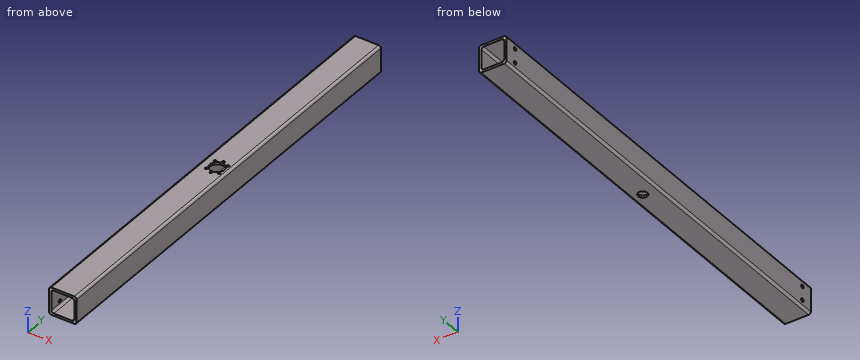
```python
from build123d import *

# Parameters (mm, degrees)
F1_DEPTH = 1226
F2_R     = 5
F3_DEPTH = 25.4
F4_R     = 3.3
F4_R_2   = 20.25
F5_DEPTH = 76.201
F6_W     = 51.969446
F6_H     = 157.89732
F6_R     = 13
F7_DEPTH = 6.35


with BuildPart() as f1:
    # F0 (on Front) → F1 (new body)
    with BuildSketch(Plane.XZ):
        with BuildLine():
            Line((50.800001, 36.691132), (-12.699999, 36.691132))
            ThreePointArc((-12.699999, 36.691132), (-17.190127, 34.83126), (-19.049999, 30.341132))
            Line((-19.049999, 30.341132), (-19.049999, -33.158868))
            ThreePointArc((-19.049999, -33.158868), (-17.190127, -37.648996), (-12.699999, -39.508868))
            Line((-12.699999, -39.508868), (50.800001, -39.508868))
            ThreePointArc((50.800001, -39.508868), (55.290129, -37.648996), (57.150001, -33.158868))
            Line((57.150001, -33.158868), (57.150001, 30.341132))
            ThreePointArc((57.150001, 30.341132), (55.290129, 34.83126), (50.800001, 36.691132))
        make_face()
        with BuildLine():
            ThreePointArc((-12.699999, 23.991132), (-10.840127, 28.48126), (-6.349999, 30.341132))
            Line((-6.349999, 30.341132), (44.450001, 30.341132))
            ThreePointArc((44.450001, 30.341132), (48.940129, 28.48126), (50.800001, 23.991132))
            Line((50.800001, 23.991132), (50.800001, -26.808868))
            ThreePointArc((50.800001, -26.808868), (48.940129, -31.298996), (44.450001, -33.158868))
            Line((44.450001, -33.158868), (-6.349999, -33.158868))
            ThreePointArc((-6.349999, -33.158868), (-10.840127, -31.298996), (-12.699999, -26.808868))
            Line((-12.699999, -26.808868), (-12.699999, 23.991132))
        make_face(mode=Mode.SUBTRACT)
    extrude(amount=F1_DEPTH)

    # F2 (on face) → F3 (cut)
    with BuildSketch(Plane(origin=(-19.049999, 0, 0), x_dir=(0, -1, 0), z_dir=(-1, 0, 0))):
        with Locations((34.062, 17.641132)):
            Circle(F2_R)
        with Locations((34.062, -20.458868)):
            Circle(F2_R)
        with Locations((1191.938, -20.458868)):
            Circle(F2_R)
        with Locations((1191.938, 17.641132)):
            Circle(F2_R)
    extrude(amount=-F3_DEPTH, mode=Mode.SUBTRACT)

    # F4 (on face) → F5 (cut, through all)
    with BuildSketch(Plane(origin=(0, 0, -39.508868), x_dir=(1, 0, 0), z_dir=(0, 0, -1))):
        with Locations((25.012778, 638.5)):
            Circle(F4_R)
        with Locations((6.981556, 631.031223)):
            Circle(F4_R)
        with Locations((6.981556, 594.968777)):
            Circle(F4_R)
        with Locations((25.012778, 587.5)):
            Circle(F4_R)
        with Locations((43.044001, 594.968777)):
            Circle(F4_R)
        with Locations((43.044001, 631.031223)):
            Circle(F4_R)
        with Locations((25.012778, 613)):
            Circle(F4_R_2)
    extrude(amount=-F5_DEPTH, mode=Mode.SUBTRACT)

    # F6 (on face) → F7 (join)
    with BuildSketch(Plane(origin=(0, 0, -39.508868), x_dir=(1, 0, 0), z_dir=(0, 0, -1))):
        with Locations((22.14342, 620.64044)):
            Rectangle(F6_W, F6_H)
        with Locations((25.012778, 613)):
            Circle(F6_R, mode=Mode.SUBTRACT)
    extrude(amount=-F7_DEPTH)


solid = f1.part
```
CAD build for the part. Positions are in the model's coordinates, mm. Coordinates: 2 decimals unless noted, no trailing zeros. Order: outer loops, then holes, each group sorted by start corner. A loop starts at its lowest first (then second) coordinate and runs counter-clockwise, first axis right, second up.
(1) Drill centre lines: L1, parallel to X at y = -613, z = 32; L2, parallel to X at y = -471, z = -4; L3, parallel to Z at x = 6, y = -413. Where is each one in solid material? Low to high.
Solution:
L1: x = -18.83 to 4.76, 45.26 to 56.93
L2: x = -19.05 to -12.7, 50.8 to 57.15
L3: z = -39.51 to -33.16, 30.34 to 36.69
(2) Saw through at A-A, the plane y = -1141. Write the cut outline in (x, z), and give its area (3 significant figures).
Solution:
outline: (-19.05, -33.16) arc R6.35 ccw to (-12.7, -39.51) - (50.8, -39.51) arc R6.35 ccw to (57.15, -33.16) - (57.15, 30.34) arc R6.35 ccw to (50.8, 36.69) - (-12.7, 36.69) arc R6.35 ccw to (-19.05, 30.34) - close; hole (-12.7, -26.81) arc R6.35 ccw to (-6.35, -33.16) - (44.45, -33.16) arc R6.35 ccw to (50.8, -26.81) - (50.8, 23.99) arc R6.35 ccw to (44.45, 30.34) - (-6.35, 30.34) arc R6.35 ccw to (-12.7, 23.99) - close
area: 1,770 mm2
(3) Pin check, flat tips, straight feed: pin 1 Ø8 at (x, z) = (26, 29) entering from -Y; pin 2 Ø9 at (y, z) = (-34.06, -20.46) entering from -X. Stop position of each tip, or through.
Solution:
pin 1: stops at y = -1226
pin 2: stops at x = 50.8
(4) Saw through at B-B, the plane z = -2. Write the cut outline in (x, y), and give its area (3 significant figures).
Solution:
outline: (-19.05, -1226) - (-12.7, -1226) - (-12.7, 0) - (-19.05, 0) - close; (50.8, -1226) - (57.15, -1226) - (57.15, 0) - (50.8, 0) - close
area: 15,600 mm2
